from build123d import *

# Parameters (mm, degrees)
EXTRUDE_1_DEPTH     = 5
SKETCH_2_W          = 20
SKETCH_2_H          = 5
CUT_EXTRUDE_1_DEPTH = 75.656062131
SKETCH_3_R          = 5.5
CUT_EXTRUDE_2_DEPTH = 75.656062131


with BuildPart() as part:
    # Эскиз1 → Бобышка-Вытянуть1 (new body)
    with BuildSketch(Plane.XY):
        with BuildLine():
            Line((-15.590383156, -64.089313216), (29.634829502, -19.482516982))
            ThreePointArc((29.634829502, -19.482516982), (31.838174922, -16.221551312), (32.612606329, -12.362939627))
            Line((32.612606329, -12.362939627), (32.612606329, 56.969735861))
            ThreePointArc((32.612606329, 56.969735861), (28.965607908, 64.692388963), (20.684732142, 66.782141332))
            Line((20.684732142, 66.782141332), (-24.540480515, 57.896601459))
            ThreePointArc((-24.540480515, 57.896601459), (-30.335259431, 54.437197567), (-32.612606329, 48.084195988))
            Line((-32.612606329, 48.084195988), (-32.612606329, -56.969735861))
            ThreePointArc((-32.612606329, -56.969735861), (-26.471218014, -66.195304454), (-15.590383156, -64.089313216))
        make_face()
    extrude(amount=EXTRUDE_1_DEPTH)

    # Эскиз2 → Вырез-Вытянуть1 (cut, through all)
    with BuildSketch(Plane.XY.offset(5)):
        with Locations((0, 34.803398117)):
            Rectangle(SKETCH_2_W, SKETCH_2_H)
        with Locations((0, 9.803398117)):
            Rectangle(SKETCH_2_W, SKETCH_2_H)
    extrude(amount=-CUT_EXTRUDE_1_DEPTH, mode=Mode.SUBTRACT)

    # Эскиз3 → Вырез-Вытянуть2 (cut, through all)
    with BuildSketch(Plane.XY.offset(5)):
        with Locations((22.612606329, 56.969735861)):
            Circle(SKETCH_3_R)
        with Locations((-22.612606329, -56.969735861)):
            Circle(SKETCH_3_R)
        with Locations((-22.612606329, 48.084195988)):
            Circle(SKETCH_3_R)
        with Locations((22.612606329, -12.362939627)):
            Circle(SKETCH_3_R)
    extrude(amount=-CUT_EXTRUDE_2_DEPTH, mode=Mode.SUBTRACT)


solid = part.part
Part model, mm, in its own coordinate system. A direction names the side the tool comes from. Give positions to 0.01 mm unless a question says otherwise; leave off trailing zeros. Loops run counter-clockwise (first coordinate to the right, second up) from the corner with the lowest first, then second, coordinate; pieces in that order, holes last.
(1) Pin check, flat tips, straight feed: pin 1 (1.5 mm diameter, centred on x = -2.5, z = 3.5, fed in from +Y); pin 2 (2.5 mm diameter, centred on x = 4, z = 2.5, fed in from -Y); pin 3 (1.5 mm diameter, centred on x = 2, z = 1.5, fed in from -Y). Stop position of each tip, or through.
Return value:
pin 1: stops at y = 62.37
pin 2: stops at y = -46
pin 3: stops at y = -47.48
(2) Band-saw the part on B-B (x = -8.5). Write the cut outline in (y, z), and give its area (3 significant figures).
Return value:
outline: (-57.1, 0) - (7.3, 0) - (7.3, 5) - (-57.1, 5) - close; (12.3, 0) - (32.3, 0) - (32.3, 5) - (12.3, 5) - close; (37.3, 0) - (61.05, 0) - (61.05, 5) - (37.3, 5) - close
area: 541 mm2
(3) Band-saw the part on C-C (y = -14.5). Write the cut outline in (x, z).
Return value:
outline: (-32.61, 0) - (17.54, 0) - (17.54, 5) - (-32.61, 5) - close; (27.68, 0) - (32.38, 0) - (32.38, 5) - (27.68, 5) - close
(4) Band-saw the part on D-D (x = 24). Write the cut outline in (y, z), and give its area (3 significant figures).
Return value:
outline: (-25.04, 0) - (-17.69, 0) - (-17.69, 5) - (-25.04, 5) - close; (-7.04, 0) - (51.65, 0) - (51.65, 5) - (-7.04, 5) - close; (62.29, 0) - (66.87, 0) - (66.87, 5) - (62.29, 5) - close
area: 353 mm2
(5) Drill centre lines: line 1 along X through (y, z) = (36, 2.7); line 2 along Y through (x, z) = (24, 4); line 3 along Y through (x, z) = (0.5, 2.05). Where is each one in solid material? Low to high.
Return value:
line 1: x = -32.61 to -10, 10 to 32.61
line 2: y = -25.04 to -17.69, -7.04 to 51.65, 62.29 to 66.87
line 3: y = -48.22 to 7.3, 12.3 to 32.3, 37.3 to 62.82
(6) Pull direction X, two halves, no side cores. Call faces 1 (the cylindrical face through (-26.62, -66.13, 2.46)), 2 (the flat face through (6.706, -42.098, 2.465)), 3 (the flat face through (-10, 35, 3)): pulls with the +X half, pulls with the -X half, needs draft (parallel to the pull), parting line crosses it, or undercut.
Return value:
face 1: parting line crosses it
face 2: pulls with the +X half
face 3: undercut
(7) 3-axis set-ups, long thin cutter, end or side, ignore diameter. For faces 4 (the flat face through (-1.61, 62.4, 2.46)), 5 (the flat face through (0, 32.303, 3)): which of +Z, -Z, +X, -X, +Y, -Y reach the whole face in a straight line?
Return value:
face 4: +Z, -Z, -X, +Y
face 5: +Z, -Z
(8) Band-saw the part on A-A (z = 2). Write the cut outline in (x, y).
Return value:
outline: (-32.61, -56.97) arc R10 ccw to (-15.59, -64.09) - (29.63, -19.48) arc R10 ccw to (32.61, -12.36) - (32.61, 56.97) arc R10 ccw to (20.68, 66.78) - (-24.54, 57.9) arc R10 ccw to (-32.61, 48.08) - close; hole circle Ø11 at (-22.61, -56.97); hole circle Ø11 at (-22.61, 48.08); hole (-10, 7.3) - (10, 7.3) - (10, 12.3) - (-10, 12.3) - close; hole (-10, 32.3) - (10, 32.3) - (10, 37.3) - (-10, 37.3) - close; hole circle Ø11 at (22.61, -12.36); hole circle Ø11 at (22.61, 56.97)
